Build history of the part. All positions in model axes, mm. A direction names the side the tool comes from. Round coordinates to 2 decimals unless told otherwise and drop trailing zeros. Write each loop counter-clockwise with the first axis right and the second up, starting at its lowest first coordinate (ties: lowest second). Pieces come first, ordered by that corner, then holes. Notation, with made-up numbers: M 39.25,7.5 L 65.25,7.5 A23 ccw 65.25,35.5 Z; hole C 20.25,38.25 d2. An arc over 180 degrees is marked long. Write item = value, one per line. Start each with the question number.
Q1. Band-saw the part on C-C on z = -40. Write the cut outline in (x, y), plus the area to 3 significant figures.
Q2. Probe L1, parallel to X at y = 4, z = -20; L2, parallel to X at y = 5.15, z = 20; L3, parallel to Y at x = -30, z = -19.5. List the from-to ranges inside material, lowest first.
Q3. Band-saw the part on D-D on y = -5. State how many separate pieces and enclosed holes the cut face has, plus the area to 3 significant figures.
Q4. Pull direction Z, two halves, no side cores. Call faces 1 (the flat face through (43, -4, 54)), 2 (the cylindrical face through (21.18, 1.48, 33.35)), 3 (the flat face through (-5, -25, 52)): released by +Z, released by -Z, zero draft, split by the parting line, or undercut.
Q5. Band-saw the part on B-B on z = 20. Write the cut outline in (x, y), plus the area to 3 significant figures.
Q6. Band-saw the part on A-A on y = -46. Write the cut outline in (x, z), plus the area to 3 significant figures.
Q7. Tool access for faces 4 (the flat face through (29.641, -20, 47)), 5 (the cylindrical face through (-1.245, 4.521, -36.998)), 6 (the cylindrical face through (43, -5, 57)): list every direction of +Z, -Z, +X, -X, +Y, -Y with a clear straight run to the whole face (end or side of a thin tool).
Q8. Drop flat-ended pins along their axis: P1, Ø3, axis at x = -28.5, y = -27.5, coming from the +Z side; P2, Ø5.5, axis at x = -40, z = 0, coming from the +Y side; P3, Ø5, axis at y = -32.5, z = 45.5, coming from the +X side; P4, Ø7.5, axis at x = 20, z = -34.64, coming from the -Y side. Give the stop position or say it passes through.
```python
from build123d import *

# Parameters (mm, degrees)
SKETCH1_R           = 45
SKETCH1_R_2         = 30
SKETCH1_R_3         = 1.75
BOSS_EXTRUDE1_DEPTH = 6
SKETCH2_R           = 36
CUT_EXTRUDE1_DEPTH  = 3
SKETCH3_R           = 3.25
CUT_EXTRUDE2_DEPTH  = 3
BOSS_EXTRUDE4_DEPTH = 6
SKETCH5_W           = 90
SKETCH5_H           = 6
BOSS_EXTRUDE6_DEPTH = 10
BOSS_EXTRUDE7_START = 50
BOSS_EXTRUDE7_DEPTH = 50
SKETCH7_W           = 29.339223388
SKETCH7_H           = 8
CUT_EXTRUDE3_DEPTH  = 114.708124382
SKETCH8_R           = 2
SKETCH8_R_2         = 1.75
CUT_EXTRUDE5_DEPTH  = 120.691269523


with BuildPart() as part:
    # Sketch1 → Boss-Extrude1 (new body)
    with BuildSketch(Plane(origin=(0, 0, 0), x_dir=(1, 0, 0), z_dir=(0, 1, 0))):
        with Locations(Location((0, 0, 0), (0, 0, 270))):
            Circle(SKETCH1_R)
        with Locations(Location((0, 0, 0), (0, 0, 270))):
            Circle(SKETCH1_R_2, mode=Mode.SUBTRACT)
        with Locations(Location((0, 40, 0), (0, 0, 270))):
            Circle(SKETCH1_R_3, mode=Mode.SUBTRACT)
        with Locations(Location((20, 34.641016151, 0), (0, 0, 270))):
            Circle(SKETCH1_R_3, mode=Mode.SUBTRACT)
        with Locations(Location((34.641016151, 20, 0), (0, 0, 270))):
            Circle(SKETCH1_R_3, mode=Mode.SUBTRACT)
        with Locations(Location((40, 0, 0), (0, 0, 270))):
            Circle(SKETCH1_R_3, mode=Mode.SUBTRACT)
        with Locations(Location((34.641016151, -20, 0), (0, 0, 270))):
            Circle(SKETCH1_R_3, mode=Mode.SUBTRACT)
        with Locations(Location((20, -34.641016151, 0), (0, 0, 270))):
            Circle(SKETCH1_R_3, mode=Mode.SUBTRACT)
        with Locations(Location((0, -40, 0), (0, 0, 270))):
            Circle(SKETCH1_R_3, mode=Mode.SUBTRACT)
        with Locations(Location((-20, -34.641016151, 0), (0, 0, 270))):
            Circle(SKETCH1_R_3, mode=Mode.SUBTRACT)
        with Locations(Location((-34.641016151, -20, 0), (0, 0, 270))):
            Circle(SKETCH1_R_3, mode=Mode.SUBTRACT)
        with Locations(Location((-40, 0, 0), (0, 0, 270))):
            Circle(SKETCH1_R_3, mode=Mode.SUBTRACT)
        with Locations(Location((-34.641016151, 20, 0), (0, 0, 270))):
            Circle(SKETCH1_R_3, mode=Mode.SUBTRACT)
        with Locations(Location((-20, 34.641016151, 0), (0, 0, 270))):
            Circle(SKETCH1_R_3, mode=Mode.SUBTRACT)
    extrude(amount=BOSS_EXTRUDE1_DEPTH)

    # Sketch2 → Cut-Extrude1 (cut)
    with BuildSketch(Plane.XZ):
        with Locations(Location((0, 0, 0), (0, 0, 270))):
            Circle(SKETCH2_R)
    extrude(amount=-CUT_EXTRUDE1_DEPTH, mode=Mode.SUBTRACT)

    # Sketch3 → Cut-Extrude2 (cut)
    with BuildSketch(Plane(origin=(0, 6, 0), x_dir=(1, 0, 0), z_dir=(0, 1, 0))):
        with Locations(Location((40, 0, 0), (0, 0, 270))):
            Circle(SKETCH3_R)
        with Locations(Location((34.641016151, -20, 0), (0, 0, 270))):
            Circle(SKETCH3_R)
        with Locations(Location((20, -34.641016151, 0), (0, 0, 270))):
            Circle(SKETCH3_R)
        with Locations(Location((0, -40, 0), (0, 0, 270))):
            Circle(SKETCH3_R)
        with Locations(Location((-20, -34.641016151, 0), (0, 0, 270))):
            Circle(SKETCH3_R)
        with Locations(Location((-34.641016151, -20, 0), (0, 0, 270))):
            Circle(SKETCH3_R)
        with Locations(Location((-40, 0, 0), (0, 0, 270))):
            Circle(SKETCH3_R)
        with Locations(Location((-34.641016151, 20, 0), (0, 0, 270))):
            Circle(SKETCH3_R)
        with Locations(Location((-20, 34.641016151, 0), (0, 0, 270))):
            Circle(SKETCH3_R)
        with Locations(Location((0, 40, 0), (0, 0, 270))):
            Circle(SKETCH3_R)
        with Locations(Location((20, 34.641016151, 0), (0, 0, 270))):
            Circle(SKETCH3_R)
        with Locations(Location((34.641016151, 20, 0), (0, 0, 270))):
            Circle(SKETCH3_R)
    extrude(amount=-CUT_EXTRUDE2_DEPTH, mode=Mode.SUBTRACT)

    # Sketch4 → Boss-Extrude4 (add)
    with BuildSketch(Plane.XZ):
        with BuildLine():
            Line((45, 0), (45, 60))
            Line((45, 60), (-45, 60))
            Line((-45, 60), (-45, 0))
            ThreePointArc((-45, 0), (0, 45), (45, 0))
        make_face()
    extrude(amount=-BOSS_EXTRUDE4_DEPTH)

    # Sketch5 → Boss-Extrude6 (add)
    with BuildSketch(Plane.XZ):
        with Locations((0, 57)):
            Rectangle(SKETCH5_W, SKETCH5_H)
    extrude(amount=BOSS_EXTRUDE6_DEPTH)

    # Sketch6 → Boss-Extrude7 (add)
    with BuildSketch(Plane.XZ.offset(BOSS_EXTRUDE7_START)):
        with BuildLine():
            Line((37.641016151, 24.660776612), (37.641016151, 60))
            Line((37.641016151, 60), (29.641016151, 60))
            Line((29.641016151, 60), (29.641016151, 33.858679264))
            ThreePointArc((29.641016151, 33.858679264), (33.953914664, 29.531875643), (37.641016151, 24.660776612))
        make_face()
        with BuildLine():
            Line((-5, 60), (5, 60))
            Line((5, 60), (5, 44.72135955))
            ThreePointArc((5, 44.72135955), (0, 45), (-5, 44.72135955))
            Line((-5, 44.72135955), (-5, 60))
        make_face()
        with BuildLine():
            Line((-29.641016151, 60), (-29.641016151, 33.858679264))
            ThreePointArc((-29.641016151, 33.858679264), (-33.953914664, 29.531875643), (-37.641016151, 24.660776612))
            Line((-37.641016151, 24.660776612), (-37.641016151, 60))
            Line((-37.641016151, 60), (-29.641016151, 60))
        make_face()
    extrude(amount=-BOSS_EXTRUDE7_DEPTH)

    # Sketch7 → Cut-Extrude3 (cut, through all)
    with BuildSketch(Plane(origin=(37.641016151, 0, 0), x_dir=(0, 0, -1), z_dir=(1, 0, 0))):
        with Locations((-39.330388306, -46)):
            Rectangle(SKETCH7_W, SKETCH7_H)
    extrude(amount=-CUT_EXTRUDE3_DEPTH, mode=Mode.SUBTRACT)

    # Sketch8 → Cut-Extrude5 (cut, through all)
    with BuildSketch(Plane(origin=(0, 0, 54), x_dir=(-1, 0, 0), z_dir=(0, 0, -1))):
        with Locations((41, -5)):
            Circle(SKETCH8_R)
        with Locations((33.641016151, -46)):
            Circle(SKETCH8_R)
        with Locations((0, -46)):
            Circle(SKETCH8_R_2)
        with Locations((15, -5)):
            Circle(SKETCH8_R_2)
        with Locations((-33.641016151, -46)):
            Circle(SKETCH8_R)
        with Locations((-41, -5)):
            Circle(SKETCH8_R)
        with Locations((-15, -5)):
            Circle(SKETCH8_R_2)
    extrude(amount=-CUT_EXTRUDE5_DEPTH, mode=Mode.SUBTRACT)


solid = part.part
```
Conclusion:
q1.outline = M -20.62,0 L -1.75,0 L -1.75,3 L -3.25,3 L -3.25,6 L -20.62,6 Z; M 1.75,0 L 20.62,0 L 20.62,6 L 3.25,6 L 3.25,3 L 1.75,3 Z
q1.area = 217 mm^2
q2.L1 = -40.31 to -37.89, -31.39 to -22.36, 22.36 to 31.39, 37.89 to 40.31
q2.L2 = -45 to -37.89, -31.39 to -22.36, 22.36 to 31.39, 37.89 to 45
q2.L3 = 3 to 6
q3.separate_pieces = 5
q3.enclosed_holes = 0
q3.area = 930 mm^2
q4.face_1 = released by -Z
q4.face_2 = undercut
q4.face_3 = zero draft
q5.outline = M -45,0 L -36.39,0 L -36.39,3 L -37.89,3 L -37.89,6 L -45,6 Z; M -32.89,0 L -29.93,0 L -29.93,3 L -22.36,3 L -22.36,6 L -31.39,6 L -31.39,3 L -32.89,3 Z; M 22.36,3 L 29.93,3 L 29.93,0 L 32.89,0 L 32.89,3 L 31.39,3 L 31.39,6 L 22.36,6 Z; M 36.39,0 L 45,0 L 45,6 L 37.89,6 L 37.89,3 L 36.39,3 Z
q5.area = 166 mm^2
q6.outline = M -37.64,54 L -35.64,54 L -35.64,60 L -37.64,60 Z; M -31.64,54 L -29.64,54 L -29.64,60 L -31.64,60 Z; M -5,54 L -1.75,54 L -1.75,60 L -5,60 Z; M 1.75,54 L 5,54 L 5,60 L 1.75,60 Z; M 29.64,54 L 31.64,54 L 31.64,60 L 29.64,60 Z; M 35.64,54 L 37.64,54 L 37.64,60 L 35.64,60 Z
q6.area = 87.0 mm^2
q7.face_4 = -Z, -Y
q7.face_5 = +Y
q7.face_6 = +Z, -Z
q8.P1 = 60
q8.P2 = 3
q8.P3 = 37.64
q8.P4 = 0
